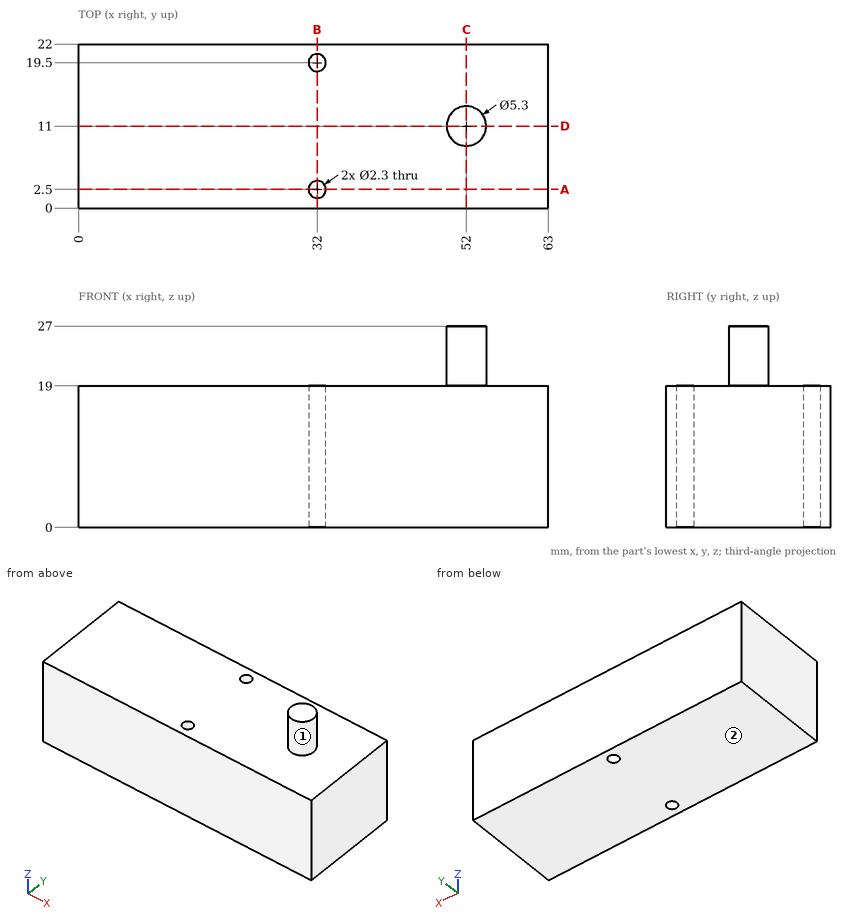
Study the drawing (mm; zero at the part's minimum x, y, z) and answer. A direction names the side the tool comes from. Give positions to 0.01 mm unless a question says otherwise; leave off trailing zeros. Loops run counter-clockwise (first coordinate to the right, second up) from the corner with the lowest first, then second, coordinate; pieces in that order, holes last. Notation, with made-up numbers: (41, 7) - (100, 7) arc R24 ccw to (100, 25) - close; hole circle Ø9 at (-16.5, 81). An arc over 180 degrees is marked (long way). Answer in a Markdown table with one row per item. Add a question column.
Q1. A tool of negligible diameter and unlimited length cuts with its end or side. For the marked faces 1 and 2, from which of +Z, -Z, +X, -X, +Y, -Y can it reach the whole face along a straight path? Write none if from no direction.
Q2. The part is cut by section D-D (y = 11). Determine the outline of the cut face in (x, z), and give its area (3 significant figures).
Q3. This flat-tipped pin is pushed along its axis until it touches: P1, Ø5, axis at x = 10.5, y = 11.5, coming from the +Z side. Where does it stop, or does it pass through?
Q4. The part is cut by section A-A (y = 2.5). Determine the outline of the cut face in (x, z), and give its area (3 significant figures).
Q5. Consider line 1 along Y through (x, z) = (32, 12.5); line 2 along Z through (x, y) = (29, 7.5); line 3 along Y through (x, z) = (32.5, 4.5). Determine where each line is inside the solid, lowest interval first.
Q6. The part is cut by section C-C (x = 52). Determine the outline of the cut face in (y, z).
Q7. The part is cut by section B-B (x = 32). Determine the outline of the cut face in (y, z), and give its area (3 significant figures).
Solution:
| question | item | result |
|---|---|---|
| 1 | face 1 | +Z |
| 1 | face 2 | -Z, +X, -X, +Y, -Y |
| 2 | outline | (0, 0) - (63, 0) - (63, 19) - (54.65, 19) - (54.65, 27) - (49.35, 27) - (49.35, 19) - (0, 19) - close |
| 2 | area | 1,240 mm² |
| 3 | P1 | stops at z = 19 |
| 4 | outline | (0, 0) - (30.85, 0) - (30.85, 19) - (0, 19) - close; (33.15, 0) - (63, 0) - (63, 19) - (33.15, 19) - close |
| 4 | area | 1,150 mm² |
| 5 | line 1 | y = 0 to 1.35, 3.65 to 18.35, 20.65 to 22 |
| 5 | line 2 | z = 0 to 19 |
| 5 | line 3 | y = 0 to 1.46, 3.54 to 18.46, 20.54 to 22 |
| 6 | outline | (0, 0) - (22, 0) - (22, 19) - (13.65, 19) - (13.65, 27) - (8.35, 27) - (8.35, 19) - (0, 19) - close |
| 7 | outline | (0, 0) - (1.35, 0) - (1.35, 19) - (0, 19) - close; (3.65, 0) - (18.35, 0) - (18.35, 19) - (3.65, 19) - close; (20.65, 0) - (22, 0) - (22, 19) - (20.65, 19) - close |
| 7 | area | 331 mm² |
